Geometry: final body of the model. Coordinates: model frame, mm. A direction names the side the tool comes from. Coordinates: 2 decimals unless noted, no trailing zeros. Write each loop counter-clockwise with the first axis right and the second up, starting at its lowest first coordinate (ties: lowest second). Pieces come first, ordered by that corner, then holes. Notation, with made-up numbers: (7.25, -20) - (32.25, -20) arc R8 ccw to (32.25, -9) - close; hole circle Ø7 at (39.25, 4). An arc over 180 degrees is marked (long way). Put each result on its own line as item: value.
```python
from build123d import *

# Parameters (mm, degrees)
SKETCH1_R           = 1.5
BOSS_EXTRUDE1_DEPTH = 3
SKETCH2_R           = 0.5
CUT_EXTRUDE1_DEPTH  = 71.099319323


with BuildPart() as part:
    # Sketch1 → Boss-Extrude1 (new body)
    with BuildSketch(Plane.XY):
        with BuildLine():
            Line((-3.585571578, 3.484777821), (25.338084336, 33.245021916))
            ThreePointArc((25.338084336, 33.245021916), (29.015202221, 34.759405952), (32.634409542, 33.111409193))
            Line((32.634409542, 33.111409193), (59.510753628, 3.351165098))
            ThreePointArc((59.510753628, 3.351165098), (60.369235466, -2.030292406), (55.8, -5))
            Line((55.8, -5), (0, -5))
            ThreePointArc((0, -5), (-4.605642686, -1.946292745), (-3.585571578, 3.484777821))
        make_face()
        with Locations((28.923655914, 29.760244095)):
            Circle(SKETCH1_R, mode=Mode.SUBTRACT)
        Circle(SKETCH1_R, mode=Mode.SUBTRACT)
        with Locations((55.8, 0)):
            Circle(SKETCH1_R, mode=Mode.SUBTRACT)
        Polygon((11.831834391, 5), (28.7897593, 22.448416138), (44.547346313, 5), align=None, mode=Mode.SUBTRACT)
    extrude(amount=BOSS_EXTRUDE1_DEPTH)

    # Sketch2 → Cut-Extrude1 (cut, through all)
    with BuildSketch(Plane.XY.offset(3)):
        with Locations((14.684404162, 14.660517535)):
            Circle(SKETCH2_R)
    extrude(amount=-CUT_EXTRUDE1_DEPTH, mode=Mode.SUBTRACT)


solid = part.part
```
1. Section query A-A (y = 0). Return loops of the section in (x, z), then the cut area to 3 significant figures.
Answer below:
outline: (-5, 0) - (-1.5, 0) - (-1.5, 3) - (-5, 3) - close; (1.5, 0) - (54.3, 0) - (54.3, 3) - (1.5, 3) - close; (57.3, 0) - (60.8, 0) - (60.8, 3) - (57.3, 3) - close
area: 179 mm²
2. Set-up query: faces 1 (the flat face through (20.19, 13.6, 1.48)), 2 (the cylindrical face through (60.4, -1.96, 1.48)). Return all of +Z, -Z, +X, -X, +Y, -Y with unobstructed straight access to the full face (end or side cutting, diameter ignored); none if empty.
Answer below:
face 1: +Z, -Z
face 2: +Z, -Z, +X
3. Section query C-C (z = 0.8). Return loops of the section in (x, y).
Answer below:
outline: (-3.59, 3.48) arc R5 ccw to (0, -5) - (55.8, -5) arc R5 ccw to (59.51, 3.35) - (32.63, 33.11) arc R5 ccw to (25.34, 33.25) - close; hole circle Ø3 at (0, 0); hole (11.83, 5) - (44.55, 5) - (28.79, 22.45) - close; hole circle Ø1 at (14.68, 14.66); hole circle Ø3 at (28.92, 29.76); hole circle Ø3 at (55.8, 0)
4. Pin query (flat end, axial travel): pin 1 Ø2.5 at (x, y) = (28.92, 29.76) entering from +Z. Return the tip coordinate at first contact, or that it passes through.
Answer below:
pin 1: passes through
5. Ray query, probe 1 along Y at (x, z) = (29, 0.3); probe 2 along X at (y, z) = (20, 1.5); probe 3 along Y at (x, z) = (14, 0.95). Return the intervals inside material, ascending. Write a range as from..to.
Answer below:
probe 1: y = -5..5, 22.22..28.26, 31.26..34.76
probe 2: x = 12.47..26.41, 31..44.48
probe 3: y = -5..5, 7.23..21.58
6. Section query B-B (y = 18). Return loops of the section in (x, z), then the cut area to 3 significant figures.
Answer below:
outline: (10.52, 0) - (24.47, 0) - (24.47, 3) - (10.52, 3) - close; (32.81, 0) - (46.28, 0) - (46.28, 3) - (32.81, 3) - close
area: 82.3 mm²
7. Section query D-D (x = 17). Return loops of the section in (y, z).
Answer below:
outline: (-5, 0) - (5, 0) - (5, 3) - (-5, 3) - close; (10.32, 0) - (24.67, 0) - (24.67, 3) - (10.32, 3) - close
8. Mould query, pull axis Y, two halves, no side actions, for faces 3 (the flat face through (10.674, 18.157, 1.479)), 4 (the flat face through (28, -5, 1)), 5 (the flat face through (36.6, 13.8, 1.5)). Classes: +Y half, -Y half, draft (parallel to the pull), parting line (faces both ways), or undercut.
Answer below:
face 3: +Y half
face 4: -Y half
face 5: undercut
